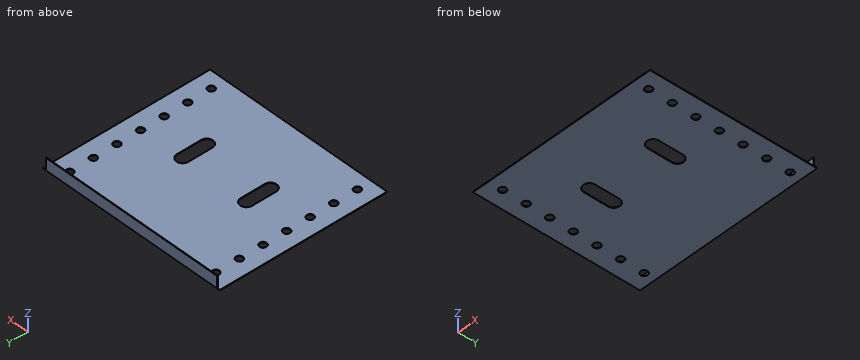
from build123d import *

# Parameters (mm, degrees)
SKETCH1_W           = 203.2
SKETCH1_H           = 177
BOSS_EXTRUDE1_DEPTH = 0.6096
CUT_EXTRUDE7_DEPTH  = 313.185220041
SKETCH4_W           = 196.85
SKETCH4_H           = 0.6096
BOSS_EXTRUDE2_DEPTH = 12
SKETCH8_R           = 3.75
CUT_EXTRUDE8_DEPTH  = 0.6096


with BuildPart() as part:
    # Sketch1 → Boss-Extrude1 (new body)
    with BuildSketch(Plane(origin=(0, 0, 0), x_dir=(1, 0, 0), z_dir=(0, 0, -1))):
        with Locations((-101.6, 148.5)):
            Rectangle(SKETCH1_W, SKETCH1_H)
    extrude(amount=BOSS_EXTRUDE1_DEPTH)

    # Sketch2 → Cut-Extrude7 (cut, through all)
    with BuildSketch(Plane(origin=(0, 0, -0.6096), x_dir=(1, 0, 0), z_dir=(0, 0, -1))):
        with BuildLine():
            Line((-131.7, 173.5), (-131.7, 148))
            ThreePointArc((-131.7, 148), (-138.2, 141.5), (-144.7, 148))
            Line((-144.7, 148), (-144.7, 173.5))
            ThreePointArc((-144.7, 173.5), (-138.2, 180), (-131.7, 173.5))
        make_face()
        with BuildLine():
            Line((-58.5, 173.5), (-58.5, 148))
            ThreePointArc((-58.5, 148), (-65, 141.5), (-71.5, 148))
            Line((-71.5, 148), (-71.5, 173.5))
            ThreePointArc((-71.5, 173.5), (-65, 180), (-58.5, 173.5))
        make_face()
    extrude(amount=-CUT_EXTRUDE7_DEPTH, mode=Mode.SUBTRACT)

    # Sketch4 → Boss-Extrude2 (add)
    with BuildSketch(Plane.XY):
        with Locations((-101.6, -60.3048)):
            Rectangle(SKETCH4_W, SKETCH4_H)
    extrude(amount=BOSS_EXTRUDE2_DEPTH)

    # Sketch8 → Cut-Extrude8 (cut)
    with BuildSketch(Plane(origin=(0, 0, -0.6096), x_dir=(-1, 0, 0), z_dir=(0, 0, -1))):
        with Locations((185.47, -222)):
            Circle(SKETCH8_R)
        with Locations((185.47, -197)):
            Circle(SKETCH8_R)
        with Locations((185.47, -172)):
            Circle(SKETCH8_R)
        with Locations((185.47, -147)):
            Circle(SKETCH8_R)
        with Locations((185.47, -122)):
            Circle(SKETCH8_R)
        with Locations((185.47, -97)):
            Circle(SKETCH8_R)
        with Locations((185.47, -72)):
            Circle(SKETCH8_R)
    cut_extrude8 = extrude(amount=-CUT_EXTRUDE8_DEPTH, mode=Mode.SUBTRACT)

    # Mirror1: Cut-Extrude8 across plane
    add(cut_extrude8.mirror(Plane(origin=(-101.6, 0, 0), x_dir=(0, 0, 1), z_dir=(1, 0, 0))), mode=Mode.SUBTRACT)


solid = part.part
Verification items for the finished model (mm, model axes). Give positions to 0.01 mm unless a question says otherwise; leave off trailing zeros. Write each loop counter-clockwise with the first axis right and the second up, starting at its lowest first coordinate (ties: lowest second). Pieces come first, ordered by that corner, then holes.
(1) Cross-section at B-B (x = -17.73). State how many separate pieces and enclosed holes the cut face has, plus the area to 3 significant figures.
(2) Gauge pin test, flat ends, axial feed: pin 1 (0.5 mm diameter, centred on y = -60, z = 3.5, fed in from +X) (3 decimals); pin 2 (3 mm diameter, centred on x = -88, y = -98, fed in from +Z); pin 3 (4 mm diameter, centred on x = -152.5, z = 8.5, fed in from -Y). Record the tip position at first contact, or that the pin passes through.
(3) Cross-section at C-C (y = -197). Enter the section's corners in (x, z), plus the area to 3 significant figures.
(4) Cross-section at A-A (x = -138.2). Enter the section's corners in (y, z), plus the area to 3 significant figures.
(5) Material ranges on line 1 (X direction, y = -197, z = -0.3); line 2 (Y direction, x = -51, z = 9.5); line 3 (Z direction, x = -141, y = -137.5), recorded low to high.
(6) Cross-section at D-D (z = 3.75). Enter the section's corners in (x, y) (3 decimals).
Worked out:
1. separate pieces: 8
1. enclosed holes: 0
1. area: 83.2 mm2
2. pin 1: stops at x = -3.175
2. pin 2: stops at z = 0
2. pin 3: stops at y = -60.61
3. outline: (-203.2, -0.61) - (-189.22, -0.61) - (-189.22, 0) - (-203.2, 0) - close; (-181.72, -0.61) - (-21.48, -0.61) - (-21.48, 0) - (-181.72, 0) - close; (-13.98, -0.61) - (0, -0.61) - (0, 0) - (-13.98, 0) - close
3. area: 115 mm2
4. outline: (-237, -0.61) - (-180, -0.61) - (-180, 0) - (-237, 0) - close; (-141.5, -0.61) - (-60, -0.61) - (-60, 12) - (-60.61, 12) - (-60.61, 0) - (-141.5, 0) - close
4. area: 91.7 mm2
5. line 1: x = -203.2 to -189.22, -181.72 to -21.48, -13.98 to 0
5. line 2: y = -60.61 to -60
5. line 3: z = -0.61 to 0
6. outline: (-200.025, -60.61) - (-3.175, -60.61) - (-3.175, -60) - (-200.025, -60) - close
